Part print with two shaded views. Sizes in mm from the minimum x, y, z corner. A direction names the side the tool comes from. Coordinates: 2 decimals unless noted, no trailing zeros. Loops run counter-clockwise (first coordinate to the right, second up) from the corner with the lowest first, then second, coordinate; pieces in that order, holes last. Notation, with made-up numbers: (41, 75.5) -> (50, 75.5) arc R13 cw to (50, 97.5) -> close; hole circle Ø7 at (-8.5, 38). An arc over 180 degrees is marked (long way). Return JSON: item names as keys, results as strings. Group by question number.
(1) Saw through at C-C on y = 45.5. Write the cut outline in (x, z), then the cut area to 3 significant figures.
(2) Saw through at B-B on x = 25. Write the cut outline in (y, z).
(3) Saw through at A-A on z = 25. Write the cut outline in (x, y).
(4) Flat gauge pins, fed straight in: pin 1 Ø2.5 at (x, z) = (45, 5) entering from +Y; pin 2 Ø5 at (x, y) = (22, 59) entering from -Z; pin 3 Ø1.5 at (x, z) = (44.5, 5) entering from -Y. Where does each tip first touch, or does it go through?
(5) Tool access for the marked faces 1 and 2: list every direction of +Z, -Z, +X, -X, +Y, -Y with a clear straight run to the whole face (end or side of a thin tool).
(6) Probe L1, parallel to Z at x = 5, y = 4.4; L2, parallel to Z at x = 45, y = 3; L3, parallel to Y at x = 13.5, z = 4.5. List the from-to ranges inside material, lowest first.
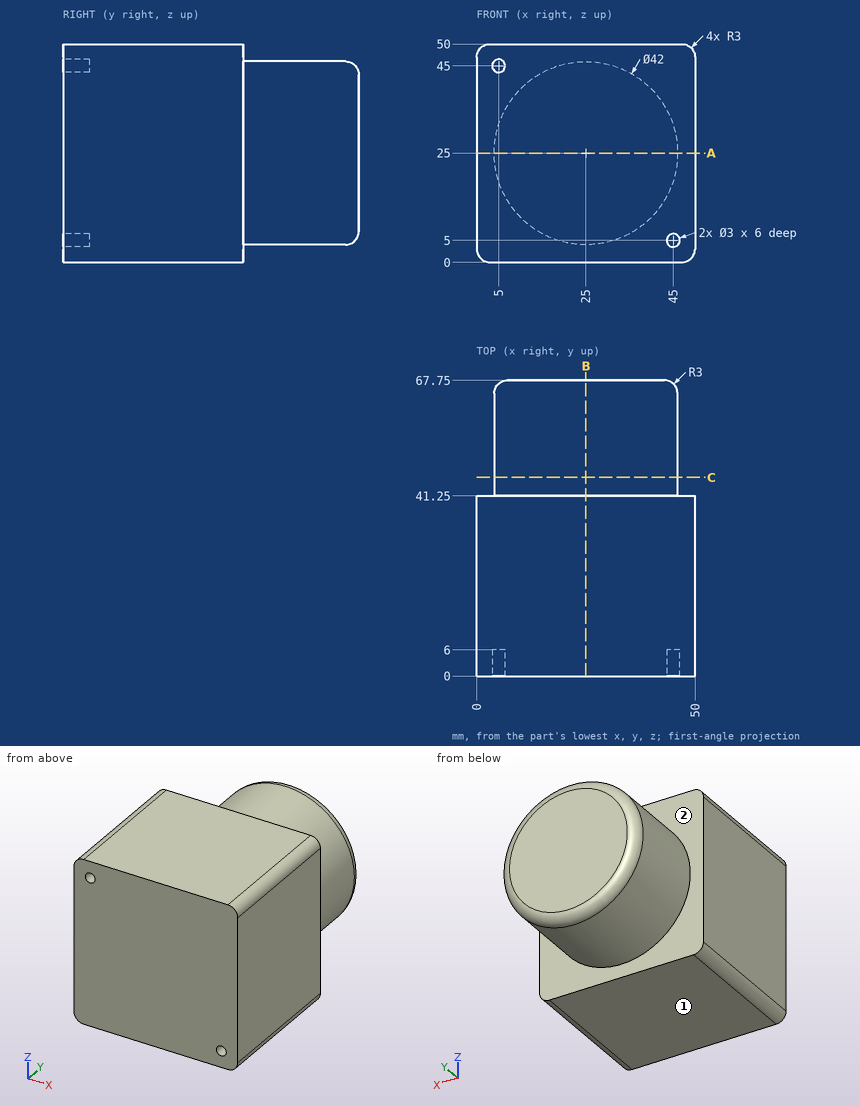
Geometry results:
{
 "1": {"outline": "circle Ø42 at (25, 25)", "area": "1,390 mm²"},
 "2": {"outline": "(0, 0) -> (41.25, 0) -> (41.25, 4) -> (64.75, 4) arc R3 ccw to (67.75, 7) -> (67.75, 43) arc R3 ccw to (64.75, 46) -> (41.25, 46) -> (41.25, 50) -> (0, 50) -> close"},
 "3": {"outline": "(0, 0) -> (50, 0) -> (50, 41.25) -> (46, 41.25) -> (46, 64.75) arc R3 ccw to (43, 67.75) -> (7, 67.75) arc R3 ccw to (4, 64.75) -> (4, 41.25) -> (0, 41.25) -> close"},
 "4": {"pin 1": "y = 41.25", "pin 2": "z = 4.01", "pin 3": "y = 6"},
 "5": {"face 1": "-Z, +X, -X, +Y, -Y", "face 2": "+Y"},
 "6": {"L1": "0 to 43.5, 46.5 to 50", "L2": "0 to 3.5, 6.5 to 50", "L3": "0 to 41.25"}
}
